Autodesk Inventor part; units mm, degrees
ref_plane "Work Plane1" through (1.525, 0, 0) normal (0, 0, 1) x (1, 0, 0)
ref_plane "YZ Plane" through (0, 0, 0) normal (1, 0, 0) x (0, 1, 0)
ref_plane "XZ Plane" through (0, 0, 0) normal (0, 1, 0) x (-1, 0, 0)
sketch "Эскиз1" plane through (0, 0, 0) normal (0, 0, 1) x (1, 0, 0)
  line L0 (0, 5) -> (70, 5)
  line L1 (70, 5) -> (70, 0)
  line L2 (70, 0) -> (0, 0)
  line L3 (-14, 0) -> (84, 0)
  line L4 (0, -1) -> (0, 6)
  line L5 (0, 5) -> (0, 0)
  dimension "d2" = 10
  dimension "d59" = 70
revolve "Базовый элемент" add sketch "Эскиз1" angle 360 about axis through (70, 0, 0) along (-1, 0, 0)
sketch "Эскиз2" plane through (0, 0, 0) normal (-1, 0, 0) x (0, 0, 1)
  line L0 (0, 9.2376) -> (8, 4.6188)
  line L1 (8, 4.6188) -> (8, -4.6188)
  line L2 (8, -4.6188) -> (0, -9.2376)
  line L3 (0, -9.2376) -> (-8, -4.6188)
  line L4 (-8, -4.6188) -> (-8, 4.6188)
  line L5 (-8, 4.6188) -> (0, 9.2376)
  line L6 (-11.2, 0) -> (11.2, 0)
  line L7 (0, 12.9326) -> (0, -12.9326)
  point P0 (0, 0)
  point P1 (0, 0)
  dimension "d11" = 16
extrude "С головкой" add sketch "Эскиз2" along normal blind 6.85
sketch "Эскиз4" plane through (0, 0, 0) normal (0, 0, 1) x (1, 0, 0)
  line L0 (-5.9262, 9.6) -> (-6.85, 8)
  line L1 (-1.1, 0) -> (-0.234, 0)
  line L2 (-8.1732, 0) -> (1.0892, 0)
  line L3 (-6.85, 9.6) -> (-5.9262, 9.6)
  line L4 (-6.85, 8) -> (-6.85, 9.6)
  line L5 (0, 11.52) -> (0, -1.92)
  dimension "d65" = 16
  dimension "d67" = 30
  dimension "d68" = 19.2
  dimension "d69" = 6.85
revolve "Фаска1" cut sketch "Эскиз4" angle 360 about axis through (-1.1, 0, 0) along (1, 0, 0)
thread "Резьба"
chamfer "Фаска2" distance 0.9202 distance2 0.9203 1 edges at (70, -5, 0) measured on face at (70, -2.0394, -1.2014)
fillet "Fillet" radius 0.4 1 edges at (0, -5, 0)
ref_plane "Work Plane1" through (1.525, 0, 0) normal (0, 0, 1) x (1, 0, 0)
equation "\"d2\" = GD"
equation "\"d59\" = NLG"
equation "\"d11\" = SW"
equation "\"d3\" = KOH"
equation "\"d71\" = RR1"
equation "\"d15\" = GEL"
equation "\"d6\" = -0.5 * SPD + 0.5 * GD"
equation "\"d65\" = SW"
equation "\"d67\" = ANG1"
equation "\"d68\" = 1.2 * SW"
equation "\"d69\" = KOH"
equation "\"NLG\" = 70"
equation "\"GD\" = NND"
equation "\"KOH\" = 6.85"
equation "\"GEL\" = 26"
equation "\"SW\" = 16"
equation "\"SW0\" = SW"
equation "\"SPD\" = NND - 1.2269 * PTC"
equation "\"SD\" = 0"
equation "\"ANG1\" = 30deg"
equation "\"GAL\" = 0.61345 * PTC"
equation "\"GUL\" = 0.61345 * PTC"
equation "\"RR\" = 0.1"
equation "\"RR1\" = 0.4"
equation "\"GD1\" = THREADDIA - 1.2269 * PTC"
equation "\"TOA\" = 30deg"
equation "\"PTC\" = 1.5"
equation "\"KOH1\" = 4.5"
equation "\"E0\" = 1.155 * SW"
properties part number "ANSI B18.2.3.5M - M10 x 1,5 x 70" material "Сталь, мягкая"
Design review of the part built by this model. Coordinates are the model's own, in mm. A direction names the side the tool comes from. Coordinates: 2 decimals unless noted, no trailing zeros. Loops run counter-clockwise (first coordinate to the right, second up) from the corner with the lowest first, then second, coordinate; pieces in that order, holes last. Notation, with made-up numbers: M 78.25,-36.75 L 96.25,-36.75 A34 ccw 96.25,-5.75 Z; hole C -35.5,-9.75 d5. An arc over 180 degrees is marked long. Answer as CSV lines item,"result".
Item 1: Add section A-A on x = 13. State the section outline as (y, z) points.
Answer list:
outline,"C 0,0 d10"
Item 2: For P1, Ø4, axis at x = 38, z = 5.5, coming from the +Y side; P2, Ø10, axis at x = 39, y = 4.5, coming from the +Z side; P3, Ø2, axis at x = 62, y = 3, coming from the -Z side; P4, Ø3, axis at x = 12.5, y = 7, coming from the +Z side, all flat-tipped, find the tip position at first contact; note any pin that passes through.
Answer list:
P1,"y = 3.57"
P2,"z = 5"
P3,"z = -4.58"
P4,"through"
Item 3: For probe 1 along Y at (x, z) = (27.5, -0.25); probe 2 along Z at (x, y) = (11, -3); probe 3 along X at (y, z) = (7.75, 0), list the stretches that pass through material, from the lowest coordinate up.
Answer list:
probe 1,"-4.99 to 4.99"
probe 2,"-4 to 4"
probe 3,"-6.85 to 0"
Item 4: Machinability: for faces 1 (the face through (70, 0, 0)), 2 (the face through (0, -4, -4)), which of the approach directions +Z, -Z, +X, -X, +Y, -Y give a long, thin tool a straight path to every point of the face, cutting with its end or side? Answer none if there is none.
Answer list:
face 1,"+Z, -Z, +X, +Y, -Y"
face 2,"+X"
